```python
from build123d import *

# Parameters (mm, degrees)
SKETCH1_R           = 1.5
BOSS_EXTRUDE1_DEPTH = 5


with BuildPart() as part:
    # Sketch1 → Boss-Extrude1 (new body)
    with BuildSketch(Plane.XY):
        with BuildLine():
            Line((-74.898979486, 5), (-4.898979486, 5))
            ThreePointArc((-4.898979486, 5), (7, 0), (-4.898979486, -5))
            Line((-4.898979486, -5), (-74.898979486, -5))
            Line((-74.898979486, -5), (-74.898979486, 5))
        make_face()
        Circle(SKETCH1_R, mode=Mode.SUBTRACT)
    extrude(amount=BOSS_EXTRUDE1_DEPTH)


solid = part.part
```
Work out the finished part from the listing and answer in its coordinate system (mm). A direction names the side the tool comes from. Give positions to 0.01 mm unless a question says otherwise; leave off trailing zeros. Order: outer loops, then holes, each group sorted by start corner. A loop starts at its lowest first (then second) coordinate and runs counter-clockwise, first axis right, second up. Notation, with made-up numbers: (64, 89.5) - (116, 89.5) arc R26 cw to (116, 122.5) - close; hole circle Ø6 at (-28, 60.5). An arc over 180 degrees is marked (long way). One line per item, written item: value. Start each with the question number.
1. Section A-A, the plane y = 0 is taken. Write down the section's boundary in (x, z), then the cut area to 3 significant figures.
2. Section B-B, the plane z = 3.3 is taken. Write down the section's boundary in (x, y).
3. Consider line 1 (Y direction, x = 0, z = 3.8); line 2 (Y direction, x = -16.5, z = 1.2); line 3 (Y direction, x = -0.5, z = 4.45). Determine where each line is inside the solid, lowest interval first.
4. Which of the six approach directions +Z, -Z, +X, -X, +Y, -Y give full straight-line access (tool end or side, diameter ignored) to faces 4 (the face through (-40, 5, 2)), 5 (the face through (-33, 0, 5))?
5. Section C-C, the plane x = 0 is taken. Write down the section's boundary in (y, z).
6. For a pull along X with two mould halves and no side action, classify faces 1 (the face through (7, 0, 2)), 2 (the face through (-1.5, 0.07, 2.46)), 3 (the face through (-39, -5, 2)) as released by +X, released by -X, zero draft, split by the parting line, or undercut.
7. This flat-tipped pin is pushed along its axis until it touches: pin 1 Ø1.5 at (x, z) = (-32.5, 2.5) entering from +Y. Where does it stop, or does it pass through?
8. Section D-D, the plane x = -20 is taken. Write down the section's boundary in (y, z), then the cut area to 3 significant figures.
Filled sheet:
1. outline: (-74.9, 0) - (-1.5, 0) - (-1.5, 5) - (-74.9, 5) - close; (1.5, 0) - (7, 0) - (7, 5) - (1.5, 5) - close
1. area: 394 mm²
2. outline: (-74.9, -5) - (-4.9, -5) arc R7 ccw (long way) to (-4.9, 5) - (-74.9, 5) - close; hole circle Ø3 at (0, 0)
3. line 1: -7 to -1.5, 1.5 to 7
3. line 2: -5 to 5
3. line 3: -6.98 to -1.41, 1.41 to 6.98
4. face 4: +Z, -Z, -X, +Y
4. face 5: +Z, +X, -X, +Y, -Y
5. outline: (-7, 0) - (-1.5, 0) - (-1.5, 5) - (-7, 5) - close; (1.5, 0) - (7, 0) - (7, 5) - (1.5, 5) - close
6. face 1: split by the parting line
6. face 2: undercut
6. face 3: zero draft
7. pin 1: y = 5
8. outline: (-5, 0) - (5, 0) - (5, 5) - (-5, 5) - close
8. area: 50.0 mm²
